from build123d import *

# Parameters (mm, degrees)
F1_DEPTH = 221.488
F3_DEPTH = 383.794
F5_DEPTH = 385.064


with BuildPart() as f1:
    # F0 (on Front) → F1 (new body)
    with BuildSketch(Plane.XZ):
        Polygon((144.416556, 169.327736), (76.817557, 120.860532), (220.943704, 120.860532), align=None)
    extrude(amount=-F1_DEPTH)

    # F2 (on Right) → F3 (cut)
    with BuildSketch(Plane.YZ):
        Polygon((-13.188886, 115.596727), (0, 121.400371), (78.753106, 175.771385), (-13.188886, 175.771385), align=None)
    extrude(amount=F3_DEPTH, mode=Mode.SUBTRACT)

    # F4 (on Right) → F5 (cut)
    with BuildSketch(Plane.YZ):
        Polygon((141.06594, 176.382303), (223.233372, 118.956745), (241.255224, 92.687599), (241.255224, 179.131404), align=None)
    extrude(amount=F5_DEPTH, mode=Mode.SUBTRACT)


solid = f1.part
The model under review builds one solid part; all positions refer to its coordinate system, in mm. Round coordinates to 2 decimals unless told otherwise and drop trailing zeros. Write each loop counter-clockwise with the first axis right and the second up, starting at its lowest first coordinate (ties: lowest second). Pieces come first, ordered by that corner, then holes. Notation, with made-up numbers: M 30,11.5 L 54,11.5 A26 cw 54,28.5 Z; hole C 16.5,86 d7. An arc over 180 degrees is marked long. Use a Markdown table: item, result. Add a question column.
Q1. We need section D-D, the plane x = 187.5. State the section outline as (y, z) points, plus the area to 3 significant figures.
Q2. Insertion check: pin 1 (3 mm diameter, centred on y = 164, z = 132.5, fed in from -X); pin 2 (2 mm diameter, centred on y = 89.5, z = 138, fed in from +X); pin 3 (1 mm diameter, centred on y = 170.5, z = 129.5, fed in from -X). Each pin has a flat end and moves straight along its axis. Give the tip position at first contact, or say it passes through.
Q3. We need section B-B, the plane y = 145. State the section outline as (x, z) points, plus the area to 3 significant figures.
Q4. We need section A-A, the plane x = 140. State the section outline as (y, z) points.
Q5. To check wall thickness, follow line 1 (Z direction, x = 110.5, y = 190.5); line 2 (X direction, y = 10.5, z = 127.5); line 3 (X direction, y = 80.5, z = 151.5). State the ranges of each line that lie inside material, in increasing order.
Q6. We need section C-C, the plane z = 142.5. State the section outline as (x, y) points, plus the area to 3 significant figures.
Findings below:
| question | item | result |
|---|---|---|
| 1 | outline | M 0,120.86 L 220.51,120.86 L 190.2,142.04 L 29.9,142.04 L 0,121.4 Z |
| 1 | area | 4,040 mm² |
| 2 | pin 1 | stops at x = 90.96 |
| 2 | pin 2 | stops at x = 195.46 |
| 2 | pin 3 | stops at x = 88.17 |
| 3 | outline | M 76.82,120.86 L 220.94,120.86 L 144.42,169.33 Z |
| 3 | area | 3,490 mm² |
| 4 | outline | M 0,120.86 L 220.51,120.86 L 155.69,166.16 L 64.83,166.16 L 0,121.4 Z |
| 5 | line 1 | z = 120.86 to 141.83 |
| 5 | line 2 | x = 86.08 to 210.46 |
| 5 | line 3 | x = 119.55 to 172.57 |
| 6 | outline | M 107,30.56 L 186.78,30.56 L 186.78,189.55 L 107,189.55 Z |
| 6 | area | 12,700 mm² |
